```python
from build123d import *

# Parameters (mm, degrees)
F2_SIZE = 0.99999


# Not quite as in the source:
# - a fillet or chamfer is up to 0.001 mm smaller than in the source, because OpenCascade refuses the exact size


with BuildPart() as f1:
    # F0 (on Front) → F1 (revolve)
    with BuildSketch(Plane.XZ):
        with BuildLine():
            Line((-8.2, -1.5365384456), (-6.2, -1.5365384456))
            Line((-6.2, -1.5365384456), (-6.2, -0.5365384456))
            ThreePointArc((-6.2, -0.5365384456), (-5.7, -0.0365384456), (-6.2, 0.4634615544))
            Line((-6.2, 0.4634615544), (-6.2, 1.4634615544))
            ThreePointArc((-6.2, 1.4634615544), (-5.7, 1.9634615544), (-6.2, 2.4634615544))
            Line((-6.2, 2.4634615544), (-6.2, 4.5634615544))
            Line((-6.2, 4.5634615544), (-3, 7.2563952203))
            Line((-3, 7.2563952203), (-3, 22))
            Line((-3, 22), (-4.566712814, 22))
            Line((-4.566712814, 22), (-5.0262918188, 16.9351019463))
            Line((-5.0262918188, 16.9351019463), (-4.4613682133, 16.7352703944))
            Line((-4.4613682133, 16.7352703944), (-4.9613682133, 12.7352703944))
            Line((-4.9613682133, 12.7352703944), (-4.4619254344, 12.7116714393))
            Line((-4.4619254344, 12.7116714393), (-5.5284631097, 7.7116714393))
            Line((-5.5284631097, 7.7116714393), (-8.2, 5.4634615544))
            Line((-8.2, 5.4634615544), (-8.2, -1.5365384456))
        make_face()
    revolve(axis=Axis((0, 0, 11), (0, 0, -1)))

    # F2 (size 1 in the source; OpenCascade refuses exactly that, so slightly less here)
    f2_edges = [f1.edges().sort_by_distance(p)[0] for p in [
        (6.2, 0, -1.536538),
    ]]
    chamfer(f2_edges, length=F2_SIZE)


solid = f1.part
```
Design review of the part built by this model. Coordinates are the model's own, in mm. A direction names the side the tool comes from. Coordinates: 2 decimals unless noted, no trailing zeros. Loops run counter-clockwise (first coordinate to the right, second up) from the corner with the lowest first, then second, coordinate; pieces in that order, holes last. Notation, with made-up numbers: (48, -11.5) - (56, -11.5) arc R19 ccw to (56, 9.5) - close; hole circle Ø9 at (-9.5, 20). An arc over 180 degrees is marked (long way). Use CSV: the item, a comma, the result in double quotes. Start each with the question number.
1) Wall thickness on L1, parallel to Y at x = 0, z = 3; L2, parallel to Z at x = 3, y = 5.25; L3, parallel to X at y = 0.75, z = 7.5: over which ranges is each line inside the solid? List them lowest first. Write a range as from..to.
2) For pin 1 Ø1.5 at (x, z) = (-4.5, 14.5) entering from +Y; pin 2 Ø9.5 at (x, y) = (0, 0) entering from -Z; pin 3 Ø2 at (y, z) = (0, 15) entering from +X, all flat-tipped, find the tip position at first contact; note any pin that passes through.
3) The part is to be moulded in two halves that separate along Y. For faces 1 (the cylindrical face through (3, 0, 15)), 2 (the cylindrical face through (1.07, 8.13, 1.91)), 3 (the flat face through (-3, -7, -1.537)), say which applies: +Y half, -Y half, draft (parallel to the pull), parting line (faces both ways), or undercut.
4) Tool access review of faces 4 (the conical face through (1.01, -4.55, 15.15)), 5 (the conical face through (-4.53, 1.43, 19.99)): name each direction out of +Z, -Z, +X, -X, +Y, -Y from which nothing blocks a thin tool from reaching the whole face with its end or side.
5) Consider section C-C on z = 3. Write out the cut boundary in (x, y), then the cut area to 3 significant figures.
6) Consider section D-D on z = 0. Write out the cut boundary in (x, y), then the cut area to 3 significant figures.
Geometry says:
1,L1,"-8.2..-6.2, 6.2..8.2"
1,L2,"-0.51..0.44, 1.49..2.44, 4.69..7.28"
1,L3,"-5.73..-2.9, 2.9..5.73"
2,pin 1,"y = 2.91"
2,pin 2,"z = 5.78"
2,pin 3,"x = 4.8"
3,face 1,"undercut"
3,face 2,"parting line"
3,face 3,"draft"
4,face 4,"none"
4,face 5,"+Z"
5,outline,"circle Ø16.4 at (0, 0); hole circle Ø12.4 at (0, 0)"
5,area,"90.5 mm^2"
6,outline,"circle Ø16.4 at (0, 0); hole circle Ø11.4 at (0, 0)"
6,area,"109 mm^2"
